from build123d import *

# Parameters (mm, degrees)
SKETCH_1_W       = 25
SKETCH_1_H       = 10
SKETCH_1_R       = 1.5
EXTRUDE_1_DEPTH  = 3
SKETCH_3_W       = 30
SKETCH_3_H       = 30
SKETCH_3_R       = 11
EXTRUDE_2_DEPTH  = 3
FILLET_START     = -1
FILLET_1_DEPTH   = 5
FILLET_1_2_DEPTH = 3
FILLET_2_R       = 5


with BuildPart() as part:
    # 草图1 → 凸台-拉伸1 (new body)
    with BuildSketch(Plane(origin=(0, 0, 0), x_dir=(1, 0, 0), z_dir=(0, 1, 0))):
        Rectangle(SKETCH_1_W, SKETCH_1_H)
        with Locations(Location((-9.5, 0, 0), (0, 0, 270))):
            Circle(SKETCH_1_R, mode=Mode.SUBTRACT)
        with Locations(Location((9.5, 0, 0), (0, 0, 270))):
            Circle(SKETCH_1_R, mode=Mode.SUBTRACT)
    extrude(amount=EXTRUDE_1_DEPTH)

    # 草图3 → 凸台-拉伸2 (add)
    with BuildSketch(Plane(origin=(0, 3, 0), x_dir=(1, 0, 0), z_dir=(0, 1, 0))):
        with Locations((0, -20)):
            Rectangle(SKETCH_3_W, SKETCH_3_H)
        with Locations(Location((0, -20, 0), (0, 0, 270))):
            Circle(SKETCH_3_R, mode=Mode.SUBTRACT)
    extrude(amount=-EXTRUDE_2_DEPTH)

    # 圆角1: read off the stored shape, not the designer's step
    # 圆角1 outline → 圆角1 (cut)
    with BuildSketch(Plane(origin=(0, 0, 0), x_dir=(1, 0, 0), z_dir=(0, 1, 0)).offset(FILLET_START)):
        with BuildLine():
            ThreePointArc((-15, -6.25), (-14.633883476, -5.366116524), (-13.75, -5))
            Line((-13.75, -5), (-15, -5))
            Line((-15, -5), (-15, -6.25))
        make_face()
        with BuildLine():
            Line((15, -5), (13.75, -5))
            ThreePointArc((13.75, -5), (14.633883476, -5.366116524), (15, -6.25))
            Line((15, -6.25), (15, -5))
        make_face()
    extrude(amount=FILLET_1_DEPTH, mode=Mode.SUBTRACT)

    # Fillet 1 2 outline → Fillet 1 2 (add)
    with BuildSketch(Plane(origin=(0, 0, 0), x_dir=(1, 0, 0), z_dir=(0, 1, 0))):
        with BuildLine():
            Line((-12.5, -5), (-12.5, -3.75))
            ThreePointArc((-12.5, -3.75), (-12.866116524, -4.633883476), (-13.75, -5))
            Line((-13.75, -5), (-12.5, -5))
        make_face()
        with BuildLine():
            ThreePointArc((13.75, -5), (12.866116524, -4.633883476), (12.5, -3.75))
            Line((12.5, -3.75), (12.5, -5))
            Line((12.5, -5), (13.75, -5))
        make_face()
    extrude(amount=FILLET_1_2_DEPTH)

    # 圆角2
    fillet_2_edges = [part.edges().sort_by_distance(p)[0] for p in [
        (-12.5, 1.5, -5),
        (12.5, 1.5, -5),
    ]]
    fillet(fillet_2_edges, radius=FILLET_2_R)


solid = part.part
Input: part model. Units: mm. Frame: model coordinates. A direction names the side the tool comes from. Coordinates: 2 decimals unless noted, no trailing zeros. Loops run counter-clockwise (first coordinate to the right, second up) from the corner with the lowest first, then second, coordinate; pieces in that order, holes last. Notation, with made-up numbers: (19.25, 21.25) - (43.25, 21.25) arc R18 ccw to (43.25, 46.25) - close; hole circle Ø6 at (4, -19). An arc over 180 degrees is marked (long way). Answer in a Markdown table with one row per item. Add a question column.
Item 1: Section query A-A on x = 0. Return the cut outline in (y, z).
Item 2: Access query for faces 4 (the cylindrical face through (-11, 1, 0)), 5 (the flat face through (-12.5, 1, 2)). Directions: +Z, -Z, +X, -X, +Y, -Y. A direction counts if a zero-diameter tool reaches every point of the face in a straight line with its end or side. Return the directions, or none.
Item 3: Mould query, pull axis Z, two halves, no side actions, for faces 1 (the cylindrical face through (-11.07, 1.52, -3.5)), 2 (the cylindrical face through (8, 1, 0)), 3 (the flat face through (12.5, 1, 2)). Classes: released by +Z, released by -Z, zero draft, split by the parting line, or undercut.
Item 4: Line query: line 1 along X through (y, z) = (1.45, 0); line 2 along X through (y, z) = (1.15, 20); line 3 along X through (y, z) = (2, 11). Output: solid intervals per line, ascending. Write a range as [from, to].
Item 5: Section query C-C on y = 2.2. Return the cut outline in (x, z), then the cut area to 3 significant figures.
Item 6: Section query B-B on z = 20. Return the cut outline in (x, y), then the cut area to 3 significant figures.
Item 7: Section query D-D on x = 9.5. Return the cut outline in (y, z), then the cut area to 3 significant figures.
Item 8: Contact query for flat-ended pins moving along their axis: P1, Ø2.5, axis at x = -9.5, z = 0, coming from the -Y side; P2, Ø5, axis at x = -7, z = 9.5, coming from the -Y side; P3, Ø1.5, axis at y = 1, z = 0.5, coming from the +X side. Output: stop coordinate, or through.
Recorded:
| question | item | result |
|---|---|---|
| 1 | outline | (0, -5) - (3, -5) - (3, 9) - (0, 9) - close; (0, 31) - (3, 31) - (3, 35) - (0, 35) - close |
| 2 | face 4 | +Y, -Y |
| 2 | face 5 | -Z, -X, +Y, -Y |
| 3 | face 1 | released by -Z |
| 3 | face 2 | undercut |
| 3 | face 3 | zero draft |
| 4 | line 1 | [-12.5, -11], [-8, 8], [11, 12.5] |
| 4 | line 2 | [-15, -11], [11, 15] |
| 4 | line 3 | [-15, -6.32], [6.32, 15] |
| 5 | outline | (-15, 6.25) arc R1.25 ccw to (-13.75, 5) arc R1.25 cw to (-12.5, 3.75) - (-12.5, 0) arc R5 ccw to (-7.5, -5) - (7.5, -5) arc R5 ccw to (12.5, 0) - (12.5, 3.75) arc R1.25 cw to (13.75, 5) arc R1.25 ccw to (15, 6.25) - (15, 35) - (-15, 35) - close; hole circle Ø3 at (-9.5, 0); hole circle Ø22 at (0, 20); hole circle Ø3 at (9.5, 0) |
| 5 | area | 745 mm^2 |
| 6 | outline | (-15, 0) - (-11, 0) - (-11, 3) - (-15, 3) - close; (11, 0) - (15, 0) - (15, 3) - (11, 3) - close |
| 6 | area | 24.0 mm^2 |
| 7 | outline | (0, -4.58) - (3, -4.58) - (3, -1.5) - (0, -1.5) - close; (0, 1.5) - (3, 1.5) - (3, 14.45) - (0, 14.45) - close; (0, 25.55) - (3, 25.55) - (3, 35) - (0, 35) - close |
| 7 | area | 76.5 mm^2 |
| 8 | P1 | through |
| 8 | P2 | y = 0 |
| 8 | P3 | x = 12.5 |
